from build123d import *

# Parameters (mm, degrees)
SKETCH1_W                      = 60
SKETCH1_H                      = 40
BOSS_EXTRUDE1_DEPTH            = 2.5
M3_CLEARANCE_HOLE1_D           = 3.4
SKETCH4_W                      = 2.5
SKETCH4_H                      = 50
BOSS_EXTRUDE2_DEPTH            = 40
FILLET1_R                      = 4
FILLET2_R                      = 1.5
CUT_EXTRUDE1_REACH             = 84.196
SKETCH6_R                      = 11
CUT_EXTRUDE1_DIRECTION_2_DEPTH = 83.196411114


with BuildPart() as part:
    # Sketch1 → Boss-Extrude1 (new body)
    with BuildSketch(Plane(origin=(0, 0, 0), x_dir=(1, 0, 0), z_dir=(0, 1, 0))):
        Rectangle(SKETCH1_W, SKETCH1_H)
    extrude(amount=BOSS_EXTRUDE1_DEPTH)

    # M3 Clearance Hole1 (through all)
    with Locations(Plane(origin=(0, 2.5, 0), x_dir=(1, 0, 0), z_dir=(0, 1, 0))):
        with Locations((-10.606601718, 10.606601718), (10.606601718, 10.606601718), (10.606601718, -10.606601718), (-10.606601718, -10.606601718)):
            Hole(M3_CLEARANCE_HOLE1_D / 2)

    # Sketch4 → Boss-Extrude2 (add)
    with BuildSketch(Plane.XY.offset(20)):
        with Locations((-28.75, 27.5)):
            Rectangle(SKETCH4_W, SKETCH4_H)
        with Locations((28.75, 27.5)):
            Rectangle(SKETCH4_W, SKETCH4_H)
    extrude(amount=-BOSS_EXTRUDE2_DEPTH)

    # Fillet1
    fillet1_edges = [part.edges().sort_by_distance(p)[0] for p in [
        (-30, 0, 0),
        (30, 0, 0),
    ]]
    fillet(fillet1_edges, radius=FILLET1_R)

    # Fillet2
    fillet2_edges = [part.edges().sort_by_distance(p)[0] for p in [
        (-27.5, 2.5, 0),
        (27.5, 2.5, 0),
    ]]
    fillet(fillet2_edges, radius=FILLET2_R)

    # Sketch6 → Cut-Extrude1 (cut, up to next)
    with BuildSketch(Plane.ZY.offset(30), mode=Mode.PRIVATE) as cut_extrude1_sk1:
        with Locations(Location((0, 31.17493075, 0), (0, 0, 180))):
            Circle(SKETCH6_R)
    cut_extrude1_tool1 = extrude(cut_extrude1_sk1.sketch, amount=-CUT_EXTRUDE1_REACH, mode=Mode.PRIVATE) & part.part
    add(cut_extrude1_tool1.solids().sort_by_distance((-30, 31.174931, 0))[0], mode=Mode.SUBTRACT)

    # Sketch6 → Cut-Extrude1 direction 2 (cut)
    with BuildSketch(Plane.ZY.offset(30)):
        with Locations(Location((0, 31.17493075, 0), (0, 0, 180))):
            Circle(SKETCH6_R)
    extrude(amount=CUT_EXTRUDE1_DIRECTION_2_DEPTH, mode=Mode.SUBTRACT)


solid = part.part
Could you check a few things on this model? Use its own coordinates, in mm. A direction names the side the tool comes from. Give positions to 0.01 mm unless a question says otherwise; leave off trailing zeros. Order: outer loops, then holes, each group sorted by start corner. A loop starts at its lowest first (then second) coordinate and runs counter-clockwise, first axis right, second up. Notation, with made-up numbers: (50, 58) - (76, 58) arc R27 cw to (76, 93) - close; hole circle Ø6 at (47.25, 71). An arc over 180 degrees is marked (long way). Return JSON: item names as keys, results as strings. Group by question number.
Q1. Which directions (+Z, -Z, +X, -X, +Y, -Y) give clear straight access to the entire face, cutting with the end or side of a thin tool? Please do faces 4 (the face through (-30, 23, 9)), 5 (the face through (0, 2.5, 0)), 6 (the face through (-28.768, 23.741, 8.107)).
Q2. Suppose I cut it at C-C, the plane y = 21. Please give me the cut outline in (x, z).
Q3. Suppose I cut it at B-B, the plane y = 15. Please give me the cut outline in (x, z).
Q4. Will this pin go through, and if not, where does the flat tip stop? pin 1 Ø6 at (x, z) = (4.5, 7.5) entering from +Y.
Q5. Please list where these lines run through material, in increasing order: line 1 along X through (y, z) = (21, -4.5); line 2 along X through (y, z) = (31.5, 8.5); line 3 along Y through (x, z) = (-10.5, -3.5). Write a range as [from, to].
Q6. Suppose I cut it at A-A, the plane z = 0. Please give me the cut outline in (x, y).
Q7. Suppose I cut it at D-D, the plane z = 17. Please give me the cut outline in (x, y).
Q8. Thinking about a two-plate mould opening in X: for faces 1 (the face through (0, 0, 0)), 2 (the face through (28.859, 1.203, -0.28)), 3 (the face through (-27.07, 2.95, -0.28)), which applies, pulls with the +X half, pulls with the -X half, needs draft (parallel to the pull), parting line crosses it, or undercut?
Resolved:
{
 "1": {"face 4": "+Z, -Z, -X, +Y, -Y", "face 5": "+Z, -Z, +Y", "face 6": "-X"},
 "2": {"outline": "(-30, -20) - (-27.5, -20) - (-27.5, -4.18) - (-30, -4.18) - close; (-30, 4.18) - (-27.5, 4.18) - (-27.5, 20) - (-30, 20) - close; (27.5, -20) - (30, -20) - (30, 20) - (27.5, 20) - close"},
 "3": {"outline": "(-30, -20) - (-27.5, -20) - (-27.5, 20) - (-30, 20) - close; (27.5, -20) - (30, -20) - (30, 20) - (27.5, 20) - close"},
 "4": {"pin 1": "stops at y = 2.5"},
 "5": {"line 1": "x = [-30, -27.5], [27.5, 30]", "line 2": "x = [27.5, 30]", "line 3": "y = [0, 2.5]"},
 "6": {"outline": "(-30, 4) arc R4 ccw to (-26, 0) - (26, 0) arc R4 ccw to (30, 4) - (30, 52.5) - (27.5, 52.5) - (27.5, 4) arc R1.5 cw to (26, 2.5) - (-26, 2.5) arc R1.5 cw to (-27.5, 4) - (-27.5, 20.17) - (-30, 20.17) - close; (-30, 42.17) - (-27.5, 42.17) - (-27.5, 52.5) - (-30, 52.5) - close"},
 "7": {"outline": "(-30, 4) arc R4 ccw to (-26, 0) - (26, 0) arc R4 ccw to (30, 4) - (30, 52.5) - (27.5, 52.5) - (27.5, 4) arc R1.5 cw to (26, 2.5) - (-26, 2.5) arc R1.5 cw to (-27.5, 4) - (-27.5, 52.5) - (-30, 52.5) - close"},
 "8": {"face 1": "needs draft", "face 2": "pulls with the +X half", "face 3": "undercut"}
}
